Source: CAD feature listing. Evaluate the final solid. Frame: model axes, mm. A direction names the side the tool comes from. Coordinates: 2 decimals unless noted, no trailing zeros. Order: outer loops, then holes, each group sorted by start corner. A loop starts at its lowest first (then second) coordinate and runs counter-clockwise, first axis right, second up. Notation, with made-up numbers: (22, -9) -> (59, -9) arc R31 ccw to (59, 19) -> close; hole circle Ø7 at (7.5, -12). An arc over 180 degrees is marked (long way). Put each result on its own line as item: value.
Autodesk Inventor part; units mm, degrees
ref_plane "YZ Plane" through (0, 0, 0) normal (1, 0, 0) x (0, 1, 0)
ref_plane "XZ Plane" through (0, 0, 0) normal (0, 1, 0) x (-1, 0, 0)
ref_plane "XY Plane" through (0, 0, 0) normal (0, 0, 1) x (1, 0, 0)
sketch "Sketch1" plane through (0, 0, 0) normal (0, 0, 1) x (1, 0, 0)
  line L0 (-6.35, -6.35) -> (6.35, -6.35)
  line L1 (6.35, -6.35) -> (6.35, 6.35)
  line L2 (6.35, 6.35) -> (-6.35, 6.35)
  line L3 (-6.35, 6.35) -> (-6.35, -6.35)
  line L4 (-6.35, -6.35) -> (6.35, 6.35) construction
  line L5 (6.35, -6.35) -> (-6.35, 6.35) construction
  line L6 (-4.7625, -4.7625) -> (4.7625, -4.7625)
  line L7 (4.7625, -4.7625) -> (4.7625, 4.7625)
  line L8 (4.7625, 4.7625) -> (-4.7625, 4.7625)
  line L9 (-4.7625, 4.7625) -> (-4.7625, -4.7625)
  line L10 (-4.7625, -4.7625) -> (4.7625, 4.7625) construction
  line L11 (4.7625, -4.7625) -> (-4.7625, 4.7625) construction
  point P0 (0, 0)
  dimension "d0" = 12.7
  dimension "d1" = 12.7
  dimension "d2" = 9.525
  dimension "d3" = 9.525
extrude "Extrusion1" add sketch "Sketch1" along normal blind 160.3375
sketch "Sketch2" plane through (6.35, -6.35, 0) normal (1, 0, 0) x (0, 0, -1)
  circle A0 centre (-118.2688, 6.35) radius 2.413
  circle A1 centre (-42.0688, 6.35) radius 2.413
  line L0 (0, 0) -> (0, 12.7)
  line L1 (-160.3375, 0) -> (-160.3375, 12.7)
  line L2 (0, 0) -> (-160.3375, 0)
  line L3 (-118.2688, 6.35) -> (-42.0688, 6.35)
  line L4 (-118.2688, 6.35) -> (-160.3375, 6.35)
  line L5 (-42.0688, 6.35) -> (0, 6.35)
  dimension "d6" = 4.826
  dimension "d7" = 4.826
  dimension "d10" = 76.2
extrude "Extrusion2" cut sketch "Sketch2" against normal blind 160.3375 contours L3 L4 A0 | A0 L4 L3 | L3 L5 A1 | A1 L5 L3
sketch "Sketch3" plane through (6.35, -6.35, 0) normal (1, 0, 0) x (0, 0, -1)
  line L0 (-160.3375, 0) -> (-160.3375, 12.7)
  line L1 (-179.3875, -12.1882) -> (-141.2875, -12.1882)
  line L2 (-141.2875, -12.1882) -> (-141.2875, 24.8882)
  line L3 (-141.2875, 24.8882) -> (-179.3875, 24.8882)
  line L4 (-179.3875, 24.8882) -> (-179.3875, -12.1882)
  line L5 (-179.3875, -12.1882) -> (-141.2875, 24.8882) construction
  line L6 (-141.2875, -12.1882) -> (-179.3875, 24.8882) construction
  line L7 (-19.05, -6.325) -> (19.05, -6.325)
  line L8 (19.05, -6.325) -> (19.05, 19.025)
  line L9 (19.05, 19.025) -> (-19.05, 19.025)
  line L10 (-19.05, 19.025) -> (-19.05, -6.325)
  line L11 (-19.05, -6.325) -> (19.05, 19.025) construction
  line L12 (19.05, -6.325) -> (-19.05, 19.025) construction
  point P0 (0, 6.35)
  point P1 (-160.3375, 6.35)
  dimension "d11" = 38.1
  dimension "d12" = 38.1
extrude "Extrusion3" cut sketch "Sketch3" against normal blind 160.3375
properties part number "box alluminum custom 6in" material "Aluminum 6061"
1. Cut plane A-A on x = 1.5. Output: boundary loops of the cut face in (y, z), plus the area to 3 significant figures.
Numbers:
outline: (-6.35, 19.05) -> (-4.76, 19.05) -> (-4.76, 141.29) -> (-6.35, 141.29) -> close; (4.76, 19.05) -> (6.35, 19.05) -> (6.35, 141.29) -> (4.76, 141.29) -> close
area: 388 mm2
2. Pull-direction query (X, two-part tool) for faces 3 (the flat face through (0, -4.762, 79)), 4 (the flat face through (6.35, 0, 79)), 5 (the cylindrical face through (-5.545, 0.725, 115.967)); classes: pulls with the +X half, pulls with the -X half, needs draft (parallel to the pull), parting line crosses it, or undercut.
Numbers:
face 3: undercut
face 4: pulls with the +X half
face 5: needs draft
3. Cut plane D-D on y = 1. Output: boundary loops of the cut face in (x, z), plus the area to 3 significant figures.
Numbers:
outline: (-6.35, 19.05) -> (-4.76, 19.05) -> (-4.76, 39.87) -> (-6.35, 39.87) -> close; (-6.35, 44.26) -> (-4.76, 44.26) -> (-4.76, 116.07) -> (-6.35, 116.07) -> close; (-6.35, 120.46) -> (-4.76, 120.46) -> (-4.76, 141.29) -> (-6.35, 141.29) -> close; (4.76, 19.05) -> (6.35, 19.05) -> (6.35, 39.87) -> (4.76, 39.87) -> close; (4.76, 44.26) -> (6.35, 44.26) -> (6.35, 116.07) -> (4.76, 116.07) -> close; (4.76, 120.46) -> (6.35, 120.46) -> (6.35, 141.29) -> (4.76, 141.29) -> close
area: 360 mm2
4. Ray query, line 1 along Z through (x, y) = (5.85, 0); line 2 along X through (y, z) = (-2.75, 94). Return the intervals inside material, ascending.
Numbers:
line 1: z = 19.05 to 39.66, 44.48 to 115.86, 120.68 to 141.29
line 2: x = -6.35 to -4.76, 4.76 to 6.35
5. Cut plane B-B on z = 30.5. Output: boundary loops of the cut face in (x, y), plus the area to 3 significant figures.
Numbers:
outline: (-6.35, -6.35) -> (6.35, -6.35) -> (6.35, 6.35) -> (-6.35, 6.35) -> close; hole (-4.76, -4.76) -> (4.76, -4.76) -> (4.76, 4.76) -> (-4.76, 4.76) -> close
area: 70.6 mm2
6. Cut plane C-C on z = 119. Output: boundary loops of the cut face in (x, y), plus the area to 3 significant figures.
Numbers:
outline: (-6.35, -6.35) -> (6.35, -6.35) -> (6.35, -2.3) -> (4.76, -2.3) -> (4.76, -4.76) -> (-4.76, -4.76) -> (-4.76, -2.3) -> (-6.35, -2.3) -> close; (-6.35, 2.3) -> (-4.76, 2.3) -> (-4.76, 4.76) -> (4.76, 4.76) -> (4.76, 2.3) -> (6.35, 2.3) -> (6.35, 6.35) -> (-6.35, 6.35) -> close
area: 56.0 mm2
7. Set-up query: faces 1 (the flat face through (-4.762, 0, 79)), 2 (the flat face through (-6.35, 0, 79)). Return all of +Z, -Z, +X, -X, +Y, -Y with unobstructed straight access to the full face (end or side cutting, diameter ignored); none if empty.
Numbers:
face 1: +Z, -Z
face 2: +Z, -Z, -X, +Y, -Y
